from build123d import *

# Parameters (mm, degrees)
F1_DEPTH    = 127
F2_T1_DEPTH = 340.4898987322
F2_T3_DEPTH = 340.4898987322


# Not quite as in the source:
# - a fillet or chamfer that OpenCascade refuses, or shapes differently, is made with other operations: its cross-section is extruded or revolved along the edge and cut away or added


with BuildPart() as f1:
    # F0 (on Front) → F1 (new body)
    with BuildSketch(Plane.XZ):
        with BuildLine():
            ThreePointArc((0, 0), (100, 64.1742430504), (200, 0))
            Line((200, 0), (201.4339410909, 2.0478801107))
            ThreePointArc((201.4339410909, 2.0478801107), (100, 65.8918877277), (-1.4339410909, 2.0478801107))
            Line((-1.4339410909, 2.0478801107), (0, 0))
        make_face()
    extrude(amount=F1_DEPTH)

    # F2: fillet of radius 33.7989898732 on 2 edges, made by hand

    # F2_s2 → F2_t1 (cut)
    with BuildSketch(Plane(origin=(-79.5992955607, 0, -113.6795752931), x_dir=(0, 1, 0), z_dir=(0.5735764364, 0, 0.8191520443))):
        with BuildLine():
            ThreePointArc((-93.2010101268, -163.8304088578), (-117.1005050634, -153.9309139212), (-127, -130.0314189846))
            Line((-127, -130.0314189846), (-127, -163.8304088578))
            Line((-127, -163.8304088578), (-93.2010101268, -163.8304088578))
        make_face()
    extrude(amount=F2_T1_DEPTH, mode=Mode.SUBTRACT)

    # F2_s4 → F2_t3 (cut)
    with BuildSketch(Plane(origin=(-49.8997015002, 0, 71.2641592346), x_dir=(0, 1, 0), z_dir=(0.5735764364, 0, -0.8191520443))):
        with BuildLine():
            ThreePointArc((-93.2010101268, 0), (-117.1005050634, 9.8994949366), (-127, 33.7989898732))
            Line((-127, 33.7989898732), (-127, 0))
            Line((-127, 0), (-93.2010101268, 0))
        make_face()
    extrude(amount=F2_T3_DEPTH, mode=Mode.SUBTRACT)


solid = f1.part
The model under review builds one solid part; all positions refer to its coordinate system, in mm. Coordinates: 2 decimals unless noted, no trailing zeros. Write each loop counter-clockwise with the first axis right and the second up, starting at its lowest first coordinate (ties: lowest second). Pieces come first, ordered by that corner, then holes. Notation, with made-up numbers: M -8,4.25 L 10,4.25 A33 ccw 10,35.25 Z; hole C 35,87 d5. An arc over 180 degrees is marked long. Put each result on its own line as item: value.
1) Add section B-B on y = -64.5. Give the boundary of the cut face in (x, z).
Computed:
outline: M -1.43,2.05 L 0,0 A110 cw 200,0 L 201.43,2.05 A112.5 ccw Z
2) Clearance check with flat-ended pins moving along their axes: pin 1 Ø1.5 at (y, z) = (-59, 46.5) entering from -X; pin 2 Ø1 at (y, z) = (-71, 35) entering from +X; pin 3 Ø1.5 at (x, y) = (148, -68) entering from +Z. State where each tip first meets the part, or that it passes through.
Computed:
pin 1: stops at x = 35.76
pin 2: stops at x = 177.96
pin 3: stops at z = 55.49
3) Wall thickness on probe 1 along Z at (x, y) = (98, -65); probe 2 along X at (y, z) = (-26, 36); probe 3 along Z at (x, y) = (113.5, -19): over which ranges is each line inside the solid? List them lowest first. Write a range as [from, to].
Computed:
probe 1: z = [64.16, 65.87]
probe 2: x = [23.63, 26.48], [173.52, 176.37]
probe 3: z = [63.34, 65.08]
4) Draft analysis for pull direction X (two halves, no side actions). For faces 1 (the cylindrical face through (98.24, -62.61, 64.16)), 2 (the cylindrical face through (101.769, -62.611, 65.878)), 3 (the cylindrical face through (3.274, -115.578, 10.089)), state which applies: released by +X, released by -X, zero draft, split by the parting line, or undercut.
Computed:
face 1: undercut
face 2: split by the parting line
face 3: released by -X
5) Add section A-A on z = 40. Give the boundary of the cut face in (x, y), then the cut area to 3 significant figures.
Computed:
outline: M 28.2,-127 L 31.2,-127 L 31.2,0 L 28.2,0 Z; M 168.8,-127 L 171.8,-127 L 171.8,0 L 168.8,0 Z
area: 761 mm2
6) Add section C-C on z = 56. Give the boundary of the cut face in (x, y), then the cut area to 3 significant figures.
Computed:
outline: M 53.87,-127 L 58.39,-127 L 58.39,0 L 53.87,0 Z; M 141.61,-127 L 146.13,-127 L 146.13,0 L 141.61,0 Z
area: 1,150 mm2
7) Add section D-D on x = 29.5. Give the boundary of the cut face in (y, z).
Computed:
outline: M -127,38.61 L 0,38.61 L 0,41.06 L -127,41.06 Z
